from build123d import *

# Parameters (mm, degrees)
SKETCH1_R           = 2
BOSS_EXTRUDE1_DEPTH = 15
SKETCH2_R           = 1.5
BOSS_EXTRUDE2_DEPTH = 10


with BuildPart() as part:
    # Sketch1 → Boss-Extrude1 (new body)
    with BuildSketch(Plane.XY):
        with BuildLine():
            Line((-16.33111253, 6.318244625), (17.66888747, 6.318244625))
            ThreePointArc((17.66888747, 6.318244625), (0.66888747, -11.07706784), (-16.33111253, 6.318244625))
        make_face()
        with Locations((0.66888747, -2.379411608)):
            Circle(SKETCH1_R, mode=Mode.SUBTRACT)
    extrude(amount=BOSS_EXTRUDE1_DEPTH)

    # Sketch2 → Boss-Extrude2 (add)
    with BuildSketch(Plane(origin=(0, 6.318244625, 0), x_dir=(1, 0, 0), z_dir=(0, 1, 0))):
        with Locations(Location((-6.33111253, -7.5, 0), (0, 0, 90))):
            Circle(SKETCH2_R)
        with Locations(Location((7.66888747, -7.5, 0), (0, 0, 90))):
            Circle(SKETCH2_R)
    extrude(amount=BOSS_EXTRUDE2_DEPTH)


solid = part.part
Model file for the job. Use its own axes, mm. A direction names the side the tool comes from. Give positions to 0.01 mm unless a question says otherwise; leave off trailing zeros. Loops run counter-clockwise (first coordinate to the right, second up) from the corner with the lowest first, then second, coordinate; pieces in that order, holes last.
Item 1: Drop flat-ended pins along their axis: P1, Ø1, axis at x = 8, y = 8, coming from the +Z side; P2, Ø3, axis at x = -4, z = 9, coming from the +Y side; P3, Ø4.5, axis at x = 3, z = 9, coming from the +Y side; P4, Ø1, axis at x = -12, z = 3.5, coming from the -Y side. Give the stop position or say it passes through.
Check values:
P1: stops at z = 9
P2: stops at y = 16.32
P3: stops at y = 6.32
P4: stops at y = -5.95
Item 2: Drill centre lines: line 1 along Y through (x, z) = (0.5, 6.25); line 2 along X through (y, z) = (-0.75, 13.5); line 3 along X through (y, z) = (-3, 8). Where is each one in solid material? Low to high.
Check values:
line 1: y = -11.08 to -4.37, -0.39 to 6.32
line 2: x = -14.97 to -0.49, 1.83 to 16.31
line 3: x = -13.8 to -1.23, 2.57 to 15.14
Item 3: Slice it at B-B (y = -2). Write the cut outline in (x, z).
Check values:
outline: (-14.37, 0) - (-1.29, 0) - (-1.29, 15) - (-14.37, 15) - close; (2.63, 0) - (15.71, 0) - (15.71, 15) - (2.63, 15) - close
Item 4: Slice it at D-D (x = -14). Write the cut outline in (y, z).
Check values:
outline: (-2.67, 0) - (6.32, 0) - (6.32, 15) - (-2.67, 15) - close
Item 5: Slice it at A-A (x = 1). Write the cut outline in (y, z).
Check values:
outline: (-11.07, 0) - (-4.35, 0) - (-4.35, 15) - (-11.07, 15) - close; (-0.41, 0) - (6.32, 0) - (6.32, 15) - (-0.41, 15) - close
Item 6: Which spindle directions (+Z, -Z, +X, -X, +Y, -Y) get a long thin tool onto all of the face, cutting with end or side? Do faces 1 (the face through (-6, 16.318, 8)), 2 (the face through (-4.867, 11.248, 7.825)). Say none if no direction does.
Check values:
face 1: +Z, -Z, +X, -X, +Y
face 2: +Y
